```python
from build123d import *

# Parameters (mm, degrees)
F1_DEPTH = 2
F3_DEPTH = 50
F4_R     = 0.99999
F5_R     = 2


# Not quite as in the source:
# - a fillet or chamfer is up to 0.001 mm smaller than in the source, because OpenCascade refuses the exact size


with BuildPart() as f1:
    # F0 (on Top) → F1 (new body)
    with BuildSketch(Plane.XY):
        with BuildLine():
            Line((-67.3099028766, 44.4781833887), (-67.3099028766, -31.5218166113))
            ThreePointArc((-67.3099028766, -31.5218166113), (-60.8662520627, -47.0781657974), (-45.3099028766, -53.5218166113))
            Line((-45.3099028766, -53.5218166113), (30.6900971234, -53.5218166113))
            ThreePointArc((30.6900971234, -53.5218166113), (46.2464463095, -47.0781657974), (52.6900971234, -31.5218166113))
            Line((52.6900971234, -31.5218166113), (52.6900971234, 44.4781833887))
            ThreePointArc((52.6900971234, 44.4781833887), (46.2464463095, 60.0345325748), (30.6900971234, 66.4781833887))
            Line((30.6900971234, 66.4781833887), (-45.3099028766, 66.4781833887))
            ThreePointArc((-45.3099028766, 66.4781833887), (-60.8662520627, 60.0345325748), (-67.3099028766, 44.4781833887))
        make_face()
        with BuildLine():
            ThreePointArc((-55.3099028766, 44.4781833887), (-52.3809706885, 51.5492512006), (-45.3099028766, 54.4781833887))
            Line((-45.3099028766, 54.4781833887), (30.6900971234, 54.4781833887))
            ThreePointArc((30.6900971234, 54.4781833887), (37.7611649352, 51.5492512006), (40.6900971234, 44.4781833887))
            Line((40.6900971234, 44.4781833887), (40.6900971234, -31.5218166113))
            ThreePointArc((40.6900971234, -31.5218166113), (37.7611649352, -38.5928844232), (30.6900971234, -41.5218166113))
            Line((30.6900971234, -41.5218166113), (-45.3099028766, -41.5218166113))
            ThreePointArc((-45.3099028766, -41.5218166113), (-52.3809706885, -38.5928844232), (-55.3099028766, -31.5218166113))
            Line((-55.3099028766, -31.5218166113), (-55.3099028766, 44.4781833887))
        make_face(mode=Mode.SUBTRACT)
    extrude(amount=F1_DEPTH)

    # F2 (on Top) → F3 (join)
    with BuildSketch(Plane.XY):
        with BuildLine():
            Line((-45.3099028766, -43.5218166113), (30.6900971234, -43.5218166113))
            ThreePointArc((30.6900971234, -43.5218166113), (39.1753784976, -40.0070979855), (42.6900971234, -31.5218166113))
            Line((42.6900971234, -31.5218166113), (42.6900971234, 44.4781833887))
            ThreePointArc((42.6900971234, 44.4781833887), (39.1753784976, 52.9634647629), (30.6900971234, 56.4781833887))
            Line((30.6900971234, 56.4781833887), (-45.3099028766, 56.4781833887))
            ThreePointArc((-45.3099028766, 56.4781833887), (-53.7951842509, 52.9634647629), (-57.3099028766, 44.4781833887))
            Line((-57.3099028766, 44.4781833887), (-57.3099028766, -31.5218166113))
            ThreePointArc((-57.3099028766, -31.5218166113), (-53.7951842509, -40.0070979855), (-45.3099028766, -43.5218166113))
        make_face()
        with BuildLine():
            Line((-45.3099028766, 54.4781833887), (30.6900971234, 54.4781833887))
            ThreePointArc((30.6900971234, 54.4781833887), (37.7611649352, 51.5492512006), (40.6900971234, 44.4781833887))
            Line((40.6900971234, 44.4781833887), (40.6900971234, -31.5218166113))
            ThreePointArc((40.6900971234, -31.5218166113), (37.7611649352, -38.5928844232), (30.6900971234, -41.5218166113))
            Line((30.6900971234, -41.5218166113), (-45.3099028766, -41.5218166113))
            ThreePointArc((-45.3099028766, -41.5218166113), (-52.3809706885, -38.5928844232), (-55.3099028766, -31.5218166113))
            Line((-55.3099028766, -31.5218166113), (-55.3099028766, 44.4781833887))
            ThreePointArc((-55.3099028766, 44.4781833887), (-52.3809706885, 51.5492512006), (-45.3099028766, 54.4781833887))
        make_face(mode=Mode.SUBTRACT)
    extrude(amount=-F3_DEPTH)

    # F4 (radius 1 in the source; OpenCascade refuses exactly that, so slightly less here)
    f4_edges = [f1.edges().sort_by_distance(p)[0] for p in [
        (-55.309903, 6.478183, -50),
        (-57.309903, 6.478183, -50),
    ]]
    fillet(f4_edges, radius=F4_R)

    # F5
    f5_edges = [f1.edges().sort_by_distance(p)[0] for p in [
        (-7.309903, 54.478183, 2),
    ]]
    fillet(f5_edges, radius=F5_R)


solid = f1.part
```
Geometry check sheet. Reference: the model listing, model coordinates, mm. A direction names the side the tool comes from. Round coordinates to 2 decimals unless told otherwise and drop trailing zeros. Write each loop counter-clockwise with the first axis right and the second up, starting at its lowest first coordinate (ties: lowest second). Pieces come first, ordered by that corner, then holes. Notation, with made-up numbers: (-20, 61) - (20, 61) arc R9 ccw to (20, 67) - close; hole circle Ø10 at (19, 1). An arc over 180 degrees is marked (long way). Write each question's results on one line, items separated by ' | '.
(1) Draft check along X on faces 1 (the face through (46.07, -47.25, 0.99)), 2 (the face through (-57.31, 7, -24)), 3 (the face through (37.68, 51.63, -24.16)), 4 (the face through (-8, -46, 2)). Enter one of: pulls with the +X half, pulls with the -X half, needs draft (parallel to the pull), parting line crosses it, or undercut.
Computed:
face 1: pulls with the +X half | face 2: pulls with the -X half | face 3: undercut | face 4: needs draft
(2) Set-up check for faces 5 (the face through (-53.7, 53.06, -24.16)), 6 (the face through (-52.303, -38.67, -24.157)), 7 (the face through (42.69, 6, -24)): record each of +Z, -Z, +X, -X, +Y, -Y from which the full face is reachable in a straight line by a thin tool's end or side.
Computed:
face 5: -Z, -X, +Y | face 6: +Z, -Z | face 7: -Z, +X, +Y, -Y
(3) Depth check by flat-ended pin: pin 1 Ø4 at (x, z) = (-10, -29.5) entering from -Y; pin 2 Ø24.5 at (x, z) = (9, -32) entering from +Y; pin 3 Ø6 at (y, z) = (39.5, -23) entering from +X. Enter the tip coordinate at first touch or a pass-through.
Computed:
pin 1: stops at y = -43.52 | pin 2: stops at y = 56.48 | pin 3: stops at x = 42.69
(4) Thickness scan on probe 1 along Y at (x, z) = (5.5, -7); probe 2 along X at (y, z) = (11.5, -44.5); probe 3 along X at (y, z) = (45.5, -26). Record the ranges inside material, lowest first. Write a range as from..to.
Computed:
probe 1: y = -43.52..-41.52, 54.48..56.48 | probe 2: x = -57.31..-55.31, 40.69..42.69 | probe 3: x = -57.27..-55.26, 40.64..42.65
(5) Sectioned sample at C-C, the plane z = -2.5. Enter the section's corners in (x, y), plus the area to 3 significant figures.
Computed:
outline: (-57.31, -31.52) arc R12 ccw to (-45.31, -43.52) - (30.69, -43.52) arc R12 ccw to (42.69, -31.52) - (42.69, 44.48) arc R12 ccw to (30.69, 56.48) - (-45.31, 56.48) arc R12 ccw to (-57.31, 44.48) - close; hole (-55.31, -31.52) arc R10 ccw to (-45.31, -41.52) - (30.69, -41.52) arc R10 ccw to (40.69, -31.52) - (40.69, 44.48) arc R10 ccw to (30.69, 54.48) - (-45.31, 54.48) arc R10 ccw to (-55.31, 44.48) - close | area: 746 mm^2
